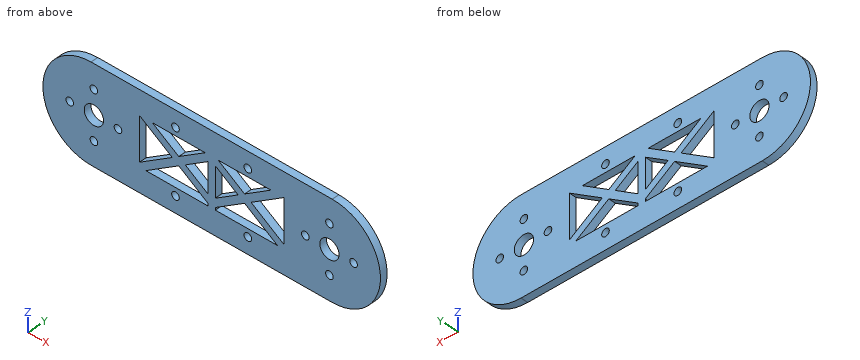
from build123d import *

# Parameters (mm, degrees)
SKETCH1_R           = 1.575
SKETCH1_R_2         = 4
BOSS_EXTRUDE1_DEPTH = 3
BOSS_EXTRUDE2_DEPTH = 3


with BuildPart() as part:
    # Sketch1 → Boss-Extrude1 (new body)
    with BuildSketch(Plane(origin=(0, 0, 0), x_dir=(1, 0, 0), z_dir=(0, 1, 0))):
        with BuildLine():
            Line((-15, 20), (-50, 20))
            ThreePointArc((-50, 20), (-70, 0), (-50, -20))
            Line((-50, -20), (50, -20))
            ThreePointArc((50, -20), (70, 0), (50, 20))
            Line((50, 20), (-15, 20))
        make_face()
        with Locations(Location((-48.85, -10, 0), (0, 0, 270))):
            Circle(SKETCH1_R, mode=Mode.SUBTRACT)
        with Locations(Location((-15, -13.25, 0), (0, 0, 270))):
            Circle(SKETCH1_R, mode=Mode.SUBTRACT)
        with BuildLine():
            ThreePointArc((-37.275, 0), (-38.85, -1.575), (-40.425, 0))
            ThreePointArc((-40.425, 0), (-38.85, 1.575), (-37.275, 0))
        make_face(mode=Mode.SUBTRACT)
        Polygon((-2.704163457, -10), (-24.591673087, -10), (-13.647918272, -2.704163457), align=None, mode=Mode.SUBTRACT)
        Polygon((-30, -10), (-30, 8.197224362), (-16.352081728, -0.901387819), align=None, mode=Mode.SUBTRACT)
        Polygon((-27.295836543, 10), (27.295836543, 10), (13.647918272, 0.901387819), (1.5, 9), (1.5, 5.394448725), (10.943754815, -0.901387819), (1.5, -7.197224362), (1.5, -10), (-1.5, -10), (-1.5, -7.197224362), (-10.943754815, -0.901387819), (-1.5, 5.394448725), (-1.5, 9), (-13.647918272, 0.901387819), align=None, mode=Mode.SUBTRACT)
        with Locations(Location((15, -13.25, 0), (0, 0, 270))):
            Circle(SKETCH1_R, mode=Mode.SUBTRACT)
        with Locations(Location((48.85, -10, 0), (0, 0, 270))):
            Circle(SKETCH1_R, mode=Mode.SUBTRACT)
        Polygon((24.591673087, -10), (2.704163457, -10), (13.647918272, -2.704163457), align=None, mode=Mode.SUBTRACT)
        Polygon((30, 8.197224362), (30, -10), (16.352081728, -0.901387819), align=None, mode=Mode.SUBTRACT)
        with Locations(Location((58.85, 0, 0), (0, 0, 270))):
            Circle(SKETCH1_R, mode=Mode.SUBTRACT)
        with Locations(Location((-58.85, 0, 0), (0, 0, 270))):
            Circle(SKETCH1_R, mode=Mode.SUBTRACT)
        with Locations(Location((-48.85, 0, 0), (0, 0, 270))):
            Circle(SKETCH1_R_2, mode=Mode.SUBTRACT)
        with Locations(Location((-48.85, 10, 0), (0, 0, 270))):
            Circle(SKETCH1_R, mode=Mode.SUBTRACT)
        with Locations(Location((-15, 13.25, 0), (0, 0, 270))):
            Circle(SKETCH1_R, mode=Mode.SUBTRACT)
        with BuildLine():
            ThreePointArc((37.275, 0), (38.85, 1.575), (40.425, 0))
            ThreePointArc((40.425, 0), (38.85, -1.575), (37.275, 0))
        make_face(mode=Mode.SUBTRACT)
        with Locations(Location((48.85, 0, 0), (0, 0, 270))):
            Circle(SKETCH1_R_2, mode=Mode.SUBTRACT)
        with Locations(Location((15, 13.25, 0), (0, 0, 270))):
            Circle(SKETCH1_R, mode=Mode.SUBTRACT)
        with Locations(Location((48.85, 10, 0), (0, 0, 270))):
            Circle(SKETCH1_R, mode=Mode.SUBTRACT)
    extrude(amount=BOSS_EXTRUDE1_DEPTH)

    # Sketch1<3> → Boss-Extrude2 (add)
    with BuildSketch(Plane(origin=(0, 0, 0), x_dir=(1, 0, 0), z_dir=(0, 1, 0))):
        Polygon((-1.5, -10), (0, -10), (0, 10), (-1.5, 9), (-1.5, 5.394448725), (-1.5, -7.197224362), align=None)
        Polygon((0, 10), (0, -10), (1.5, -10), (1.5, -7.197224362), (1.5, 5.394448725), (1.5, 9), align=None)
        Polygon((1.5, 10), (0, 10), (1.5, 9), align=None)
        Polygon((-1.5, 9), (0, 10), (-1.5, 10), align=None)
    extrude(amount=BOSS_EXTRUDE2_DEPTH)


solid = part.part
Verification items for the finished model (mm, model axes). Coordinates: 2 decimals unless noted, no trailing zeros. Loops run counter-clockwise (first coordinate to the right, second up) from the corner with the lowest first, then second, coordinate; pieces in that order, holes last. Notation, with made-up numbers: (15, 3) -> (36, 3) arc R18 ccw to (36, 10) -> close; hole circle Ø3 at (53.5, -14.5). An arc over 180 degrees is marked (long way). Answer as a JSON object with one key per item and string values. Group by question number.
Item 1: Scan lines: probe 1 along Z at (x, y) = (-4.5, 2.1); probe 2 along X at (y, z) = (1.2, 8); probe 3 along X at (y, z) = (1.9, -12). Record each from-to range of solid material in increasing order.
Item 2: Sectioned sample at C-C on x = 15. Record the boundary of the cut face in (y, z) (3 decimals).
Item 3: Sectioned sample at D-D on y = 1.15. State how many separate pieces and enclosed holes the cut face has, plus the area to 3 significant figures.
Item 4: Sectioned sample at B-B on z = 13.25. Record the boundary of the cut face in (x, y) (3 decimals).
Item 5: Sectioned sample at A-A on x = 38.85. Record the boundary of the cut face in (y, z) (3 decimals).
Item 6: Depth check by flat-ended pin: pin 1 (3.5 mm diameter, centred on x = 58.85, z = 0, fed in from -Y); pin 2 (1.5 mm diameter, centred on y = 2, z = 14.5, fed in from +X); pin 3 (1.5 mm diameter, centred on y = 2.5, z = 10, fed in from +X); pin 4 (3 mm diameter, centred on x = 15, z = 13.25, fed in from +Y). Enter the tip coordinate at first touch or a pass-through.
Evaluation:
{
 "1": {"probe 1": "z = -20 to -10, -7 to -3.39, 5.2 to 8.8, 10 to 20", "probe 2": "x = -68.33 to -30, -27 to -21.59, -5.7 to 5.7, 21.59 to 27, 30 to 68.33", "probe 3": "x = -66 to -15.96, -14.04 to 14.04, 15.96 to 66"},
 "2": {"outline": "(0, -20) -> (3, -20) -> (3, -14.825) -> (0, -14.825) -> close; (0, -11.675) -> (3, -11.675) -> (3, -10) -> (0, -10) -> close; (0, -1.803) -> (3, -1.803) -> (3, 3.606) -> (0, 3.606) -> close; (0, 10) -> (3, 10) -> (3, 11.675) -> (0, 11.675) -> close; (0, 14.825) -> (3, 14.825) -> (3, 20) -> (0, 20) -> close"},
 "3": {"separate pieces": "1", "enclosed holes": "22", "area": "4,290 mm²"},
 "4": {"outline": "(-64.981, 0) -> (-16.575, 0) -> (-16.575, 3) -> (-64.981, 3) -> close; (-13.425, 0) -> (13.425, 0) -> (13.425, 3) -> (-13.425, 3) -> close; (16.575, 0) -> (64.981, 0) -> (64.981, 3) -> (16.575, 3) -> close"},
 "5": {"outline": "(0, -20) -> (3, -20) -> (3, -1.575) -> (0, -1.575) -> close; (0, 1.575) -> (3, 1.575) -> (3, 20) -> (0, 20) -> close"},
 "6": {"pin 1": "stops at y = 0", "pin 2": "stops at x = 64.52", "pin 3": "stops at x = 67.73", "pin 4": "passes through"}
}
